Read the model definition and answer for the solid it produces. Units are mm, in the model's axes. A direction names the side the tool comes from. Coordinates: 2 decimals unless noted, no trailing zeros. Order: outer loops, then holes, each group sorted by start corner. A loop starts at its lowest first (then second) coordinate and runs counter-clockwise, first axis right, second up.
from build123d import *

# Parameters (mm, degrees)
EXTRUDE_2_DEPTH     = 20
SKETCH_10_R         = 3
CUT_EXTRUDE_1_DEPTH = 214.072757527
SKETCH_11_R         = 3
CUT_EXTRUDE_2_DEPTH = 214.072757527


with BuildPart() as part:
    # 草图9 → 凸台-拉伸2 (new body)
    with BuildSketch(Plane.XY):
        with BuildLine():
            Line((-150, 0), (-110.203390468, 66.224778592))
            ThreePointArc((-110.203390468, 66.224778592), (-32.188335395, 124.476582676), (64.285512696, 111.345774179))
            Line((64.285512696, 111.345774179), (64.285512696, 29.910799468))
            Line((64.285512696, 29.910799468), (73.817743163, 29.910799468))
            Line((73.817743163, 29.910799468), (75, 129.903810568))
            ThreePointArc((75, 129.903810568), (-75, 129.903810568), (-150, 0))
        make_face()
    extrude(amount=EXTRUDE_2_DEPTH)

    # 草图10 → 切除-拉伸1 (cut, through all)
    with BuildSketch(Plane.XY.offset(20)):
        with Locations((69.588650595, 126.928706674)):
            Circle(SKETCH_10_R)
    extrude(amount=-CUT_EXTRUDE_1_DEPTH, mode=Mode.SUBTRACT)

    # 草图11 → 切除-拉伸2 (cut, through all)
    with BuildSketch(Plane.XY.offset(20)):
        with Locations((69.114412229, 34.162597533)):
            Circle(SKETCH_11_R)
    extrude(amount=-CUT_EXTRUDE_2_DEPTH, mode=Mode.SUBTRACT)


solid = part.part
Q1. The part is cut by section A-A, the plane y = 63. Determine the outline of the cut face in (x, z), then the cut area to 3 significant figures.
Q2. The part is cut by section C-C, the plane y = 105.5. Determine the outline of the cut face in (x, z).
Q3. The part is cut by section B-B, the plane z = 16.5. Determine the outline of the cut face in (x, y), then the cut area to 3 significant figures.
Q4. Which of the six approach directions +Z, -Z, +X, -X, +Y, -Y give full straight-line access (tool end or side, diameter ignored) to faces 5 (the flat face through (69, 29.911, 10)), 6 (the flat face through (-130.38, 32.65, 9.86)), 7 (the flat face through (-38, 125, 20))?
Q5. Each of these flat-tipped pins is pushed along its axis until it touches: P1, Ø2, axis at x = -75.5, z = 5, coming from the +Y side; P2, Ø1.5, axis at y = 115, z = 12.5, coming from the -X side; P3, Ø6, axis at y = 60, z = 6, coming from the -X side; P4, Ø5, axis at x = 69.59, y = 126.93, coming from the +Z side. Where does it stop, or does it pass through?
Q6. The part is cut by section D-D, the plane x = -100.5. Determine the outline of the cut face in (y, z), then the cut area to 3 significant figures.
Q7. Determine the mould class of faces 1 (the cylindrical face through (66.117, 34.295, 10.14)), 2 (the flat face through (64.286, 71, 10)), 3 (the cylindrical face through (-73.09, 130.99, 9.86)), 4 (the cylindrical face through (-33.54, 124.12, 9.86)) for opening direction Y: +Y half, -Y half, draft (parallel to the pull), parting line (faces both ways), or undercut.
Q8. Straight lines are drawn through the part: L1, parallel to X at y = 35.5, z = 6.5; L2, parallel to X at y = 114, z = 11.75; L3, parallel to X at y = 84, z = 18. For each, find the intervals that lie inside material, in ascending order.
Computed values:
1. outline: (-136.13, 0) - (-112.14, 0) - (-112.14, 20) - (-136.13, 20) - close; (64.29, 0) - (74.21, 0) - (74.21, 20) - (64.29, 20) - close
1. area: 678 mm2
2. outline: (-106.63, 0) - (-73.49, 0) - (-73.49, 20) - (-106.63, 20) - close; (64.29, 0) - (74.71, 0) - (74.71, 20) - (64.29, 20) - close
3. outline: (-150, 0) - (-110.2, 66.22) arc R128.57 cw to (64.29, 111.35) - (64.29, 29.91) - (73.82, 29.91) - (75, 129.9) arc R150 ccw to start; hole circle Ø6 at (69.11, 34.16); hole circle Ø6 at (69.59, 126.93)
3. area: 6,610 mm2
4. face 5: +Z, -Z, +X, -Y
4. face 6: +Z, -Z, -Y
4. face 7: +Z, +X, -X, +Y, -Y
5. P1: stops at y = 130.19
5. P2: stops at x = -97.2
5. P3: stops at x = -138.75
5. P4: passes through
6. outline: (80.19, 0) - (111.35, 0) - (111.35, 20) - (80.19, 20) - close
6. area: 623 mm2
7. face 1: undercut
7. face 2: draft
7. face 3: +Y half
7. face 4: -Y half
8. L1: x = -145.74 to -128.67, 64.29 to 66.43, 71.8 to 73.88
8. L2: x = -97.49 to -59.45, 59.45 to 74.81
8. L3: x = -124.27 to -97.34, 64.29 to 74.46
